from build123d import *

# Parameters (mm, degrees)
F1_DEPTH = 20
F3_DEPTH = 40
F5_DEPTH = 40
F6_R     = 2
F7_DEPTH = 50
F8_R     = 2
F9_DEPTH = 50


with BuildPart() as f1:
    # F0 (on Front) → F1 (new body, symmetric)
    with BuildSketch(Plane.XZ):
        Polygon((0, 40), (0, 0), (40, 0), (40, 10), (10, 40), align=None)
    extrude(amount=F1_DEPTH, both=True)

    # F2 (on face) → F3 (join)
    with BuildSketch(Plane(origin=(0, 0, 0), x_dir=(0, -1, 0), z_dir=(-1, 0, 0))):
        with BuildLine():
            ThreePointArc((-8, 0), (0, -8), (8, 0))
            Line((8, 0), (-8, 0))
        make_face()
    extrude(amount=-F3_DEPTH)

    # F4 (on face) → F5 (join)
    with BuildSketch(Plane(origin=(0, 0, 0), x_dir=(1, 0, 0), z_dir=(0, 0, -1))):
        with BuildLine():
            ThreePointArc((0, -8), (5.6568542495, -5.6568542495), (8, 0))
            ThreePointArc((8, 0), (5.6568542495, 5.6568542495), (0, 8))
            ThreePointArc((0, 8), (-8, 0), (0, -8))
        make_face()
    extrude(amount=-F5_DEPTH)

    # F6 (on face) → F7 (cut, symmetric)
    with BuildSketch(Plane(origin=(0, 0, 0), x_dir=(0, -1, 0), z_dir=(-1, 0, 0))):
        with Locations((0, 25)):
            Circle(F6_R)
    extrude(amount=F7_DEPTH, both=True, mode=Mode.SUBTRACT)

    # F8 (on face) → F9 (cut, symmetric)
    with BuildSketch(Plane(origin=(0, 0, 0), x_dir=(1, 0, 0), z_dir=(0, 0, -1))):
        with Locations((25, 0)):
            Circle(F8_R)
    extrude(amount=F9_DEPTH, both=True, mode=Mode.SUBTRACT)


solid = f1.part
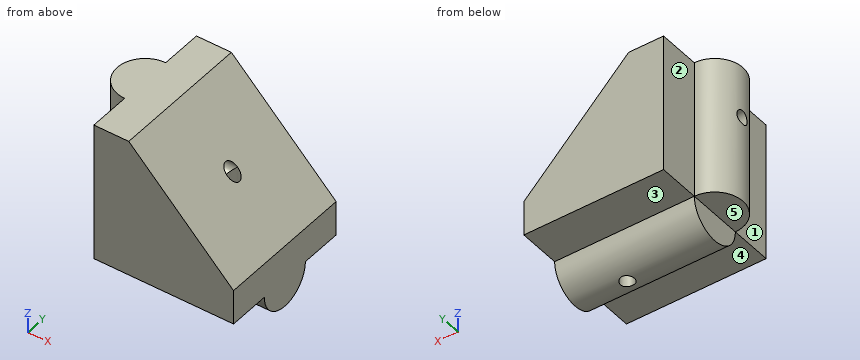
Geometry: final body of the model. Coordinates: model frame, mm. Face numbers are marked on the shaded views. A direction names the side the tool comes from. Give positions to 0.01 mm unless a question says otherwise; leave off trailing zeros. Loops run counter-clockwise (first coordinate to the right, second up) from the corner with the lowest first, then second, coordinate; pieces in that order, holes last. Notation, with made-up numbers: (76.5, 57) -> (85.5, 57) arc R9 cw to (85.5, 72) -> close; hole circle Ø6 at (3, 35). An arc over 180 degrees is marked (long way). Put each result on its own line as item: value.
1. Cut plane C-C (x = 14.5). Return the cut outline in (y, z), plus the area to 3 significant figures.
Taken from the geometry:
outline: (-20, 0) -> (-8, 0) arc R8 ccw to (8, 0) -> (20, 0) -> (20, 35.5) -> (-20, 35.5) -> close; hole circle Ø4 at (0, 25)
area: 1,510 mm2
2. Cut plane A-A (z = 1.5). Return the cut outline in (x, y), plus the area to 3 significant figures.
Taken from the geometry:
outline: (0, -20) -> (40, -20) -> (40, 20) -> (0, 20) -> (0, 8) arc R8 ccw to (0, -8) -> close; hole circle Ø4 at (25, 0)
area: 1,690 mm2
3. Cut plane D-D (y = -12). Return the cut outline in (x, z).
Taken from the geometry:
outline: (0, 0) -> (40, 0) -> (40, 10) -> (10, 40) -> (0, 40) -> close
4. Ray query, line 1 along Y through (x, z) = (14, 25); line 2 along Z through (x, y) = (8.5, 0); line 3 along Y through (x, z) = (24, 1.5). Return the intervals inside material, ascending. Write a range as [from, to].
Taken from the geometry:
line 1: y = [-20, -2], [2, 20]
line 2: z = [-8, 23], [27, 40]
line 3: y = [-20, -1.73], [1.73, 20]
5. Set-up query: the marked faces 1, 2, 3, 4 and 5. Return all of +Z, -Z, +X, -X, +Y, -Y with unobstructed straight access to the full face (end or side cutting, diameter ignored); none if empty.
Taken from the geometry:
face 1: +Z, -Z, -X, -Y
face 2: +Z, -Z, -X, +Y
face 3: -Z, +X, -X, +Y
face 4: -Z, +X, -X, -Y
face 5: -Z, -X, +Y, -Y
6. Pin query (flat end, axial travel): P1, Ø9.5, axis at x = 18.5, y = 16.5, coming from the -Z side; P2, Ø9.5, axis at y = 14.5, z = 16, coming from the -X side; P3, Ø5, axis at x = 18.5, y = 1.5, coming from the +Z side. Return the tip coordinate at first contact, or that it passes through.
Taken from the geometry:
P1: stops at z = 0
P2: stops at x = 0
P3: stops at z = 34
7. Cut plane B-B (y = 0). Return the cut outline in (x, z), plus the area to 3 significant figures.
Taken from the geometry:
outline: (-8, 0) -> (0, 0) -> (0, -8) -> (23, -8) -> (23, 23) -> (-8, 23) -> close; (-8, 27) -> (23, 27) -> (10, 40) -> (-8, 40) -> close; (27, -8) -> (40, -8) -> (40, 10) -> (27, 23) -> close
area: 1,530 mm2
